Geometry check sheet. Reference: the model listing, model coordinates, mm. A direction names the side the tool comes from. Give positions to 0.01 mm unless a question says otherwise; leave off trailing zeros. Loops run counter-clockwise (first coordinate to the right, second up) from the corner with the lowest first, then second, coordinate; pieces in that order, holes last.
1. Cross-section at B-B, the plane z = -13. Record the cut outline in (x, y).
2. Cross-section at A-A, the plane x = -35.5. Record the cut outline in (y, z), plus the area to 3 significant figures.
3. Material ranges on L1, parallel to X at y = 33.5, z = -2.25; L2, parallel to Z at x = -31.5, y = -12.5; L3, parallel to Y at x = -6.5, z = 2, recorded low to high.
4. Cross-section at C-C, the plane x = 0. Record the cut outline in (y, z).
5. Go/stop test with flat-tipped pins: pin 1 Ø14 at (x, y) = (-20, 22) entering from -Z; pin 2 Ø4 at (x, z) = (0, -4.5) entering from +Y; pin 3 Ø6.5 at (x, y) = (-24, 35) entering from -Z; pin 4 Ø3.5 at (x, y) = (-34.04, -21.19) entering from +Z. Record where each tip stops, or that it passes through.
6. Tool access check on faces 1 (the cylindrical face through (-3, 0, 6)), 2 (the flat face through (-33.4, 7.85, 2.46)), 3 (the cylindrical face through (-26.389, 35.757, -2.535)). Record the directions out of +Z, -Z, +X, -X, +Y, -Y that give a thin tool (end or side, any length) a straight path to the whole face; none if there is none.
7. Cross-section at D-D, the plane y = 0. Record the cut outline in (x, z), plus the area to 3 significant figures.
8. Release check for a two-part mould opening along Y. For faces 4 (the cylindrical face through (-3, 0, -9)), 5 (the cylindrical face through (-36.25, -19.16, 2.46)), 6 (the flat face through (0, 0, 8)) record: +Y half, -Y half, draft (parallel to the pull), parting line (faces both ways), or undercut.
from build123d import *

# Parameters (mm, degrees)
SKETCH1_R           = 3
BOSS_EXTRUDE1_DEPTH = 5
BOSS_EXTRUDE2_START = -10
SKETCH2_R           = 3
BOSS_EXTRUDE2_DEPTH = 10
BOSS_EXTRUDE3_START = -22
SKETCH3_R           = 3
BOSS_EXTRUDE3_DEPTH = 22
SKETCH4_R           = 3
BOSS_EXTRUDE4_DEPTH = 3


with BuildPart() as part:
    # Sketch1 → Boss-Extrude1 (new body)
    with BuildSketch(Plane.XY):
        Polygon((-26.724502293, 45.005919314), (-40.262558922, -30.363907626), (6.455683288, -1.282016359), align=None)
        with Locations((-24.177985347, 33.729438545)):
            Circle(SKETCH1_R, mode=Mode.SUBTRACT)
        Circle(SKETCH1_R, mode=Mode.SUBTRACT)
        with Locations((-34.042997525, -21.191609649)):
            Circle(SKETCH1_R, mode=Mode.SUBTRACT)
    extrude(amount=BOSS_EXTRUDE1_DEPTH)

    # Sketch2 → Boss-Extrude2 (add)
    with BuildSketch(Plane.XY.offset(5).offset(BOSS_EXTRUDE2_START)):
        with Locations((-24.177985347, 33.729438545)):
            Circle(SKETCH2_R)
    extrude(amount=BOSS_EXTRUDE2_DEPTH)

    # Sketch3 → Boss-Extrude3 (add)
    with BuildSketch(Plane.XY.offset(5).offset(BOSS_EXTRUDE3_START)):
        Circle(SKETCH3_R)
    extrude(amount=BOSS_EXTRUDE3_DEPTH)

    # Sketch4 → Boss-Extrude4 (add)
    with BuildSketch(Plane.XY.offset(5)):
        Circle(SKETCH4_R)
    extrude(amount=BOSS_EXTRUDE4_DEPTH)


solid = part.part
Result:
1. outline: circle Ø6 at (0, 0)
2. outline: (-27.4, 0) - (-23.81, 0) - (-23.81, 5) - (-27.4, 5) - close; (-18.57, 0) - (-3.85, 0) - (-3.85, 5) - (-18.57, 5) - close
2. area: 91.5 mm2
3. L1: x = -27.17 to -21.19
3. L2: z = 0 to 5
3. L3: y = -9.35 to 16.79
4. outline: (-5.3, 0) - (-3, 0) - (-3, -17) - (3, -17) - (3, 0) - (7.72, 0) - (7.72, 5) - (3, 5) - (3, 8) - (-3, 8) - (-3, 5) - (-5.3, 5) - close
5. pin 1: stops at z = 0
5. pin 2: stops at y = 3
5. pin 3: stops at z = -5
5. pin 4: passes through
6. face 1: +Z
6. face 2: +Z, -Z, -X, +Y
6. face 3: -Z
7. outline: (-34.81, 0) - (-3, 0) - (-3, -17) - (3, -17) - (3, 0) - (5.54, 0) - (5.54, 5) - (3, 5) - (3, 8) - (-3, 8) - (-3, 5) - (-34.81, 5) - close
7. area: 322 mm2
8. face 4: parting line
8. face 5: undercut
8. face 6: draft
